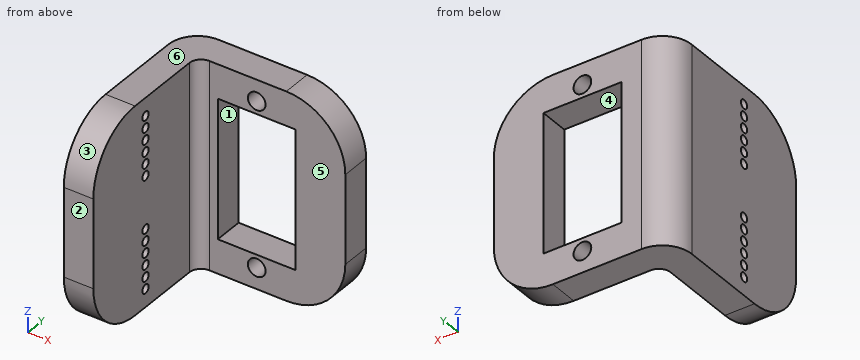
from build123d import *

# Parameters (mm, degrees)
SKETCH1_W           = 35
SKETCH1_H           = 25
SKETCH1_R           = 0.75
BOSS_EXTRUDE1_DEPTH = 5
SKETCH4_W           = 30
SKETCH4_H           = 35
BOSS_EXTRUDE2_DEPTH = 5
CUT_EXTRUDE2_REACH  = 47.894
SKETCH3_R           = 1.5
SKETCH3_W           = 23.5
SKETCH3_H           = 13.2
FILLET1_R           = 10
FILLET2_R           = 5
FILLET3_R           = 2
FILLET4_R           = 10


with BuildPart() as part:
    # Sketch1 → Boss-Extrude1 (new body)
    with BuildSketch(Plane(origin=(0, 0, 0), x_dir=(0, 0, -1), z_dir=(1, 0, 0))):
        Rectangle(SKETCH1_W, SKETCH1_H)
        with Locations((-14.45, 0)):
            Circle(SKETCH1_R, mode=Mode.SUBTRACT)
        with Locations((-12.45, 0)):
            Circle(SKETCH1_R, mode=Mode.SUBTRACT)
        with Locations((-10.45, 0)):
            Circle(SKETCH1_R, mode=Mode.SUBTRACT)
        with Locations((-8.45, 0)):
            Circle(SKETCH1_R, mode=Mode.SUBTRACT)
        with Locations((-6.45, 0)):
            Circle(SKETCH1_R, mode=Mode.SUBTRACT)
        with Locations((-4.45, 0)):
            Circle(SKETCH1_R, mode=Mode.SUBTRACT)
        with Locations((4.45, 0)):
            Circle(SKETCH1_R, mode=Mode.SUBTRACT)
        with Locations((6.45, 0)):
            Circle(SKETCH1_R, mode=Mode.SUBTRACT)
        with Locations((8.45, 0)):
            Circle(SKETCH1_R, mode=Mode.SUBTRACT)
        with Locations((10.45, 0)):
            Circle(SKETCH1_R, mode=Mode.SUBTRACT)
        with Locations((12.45, 0)):
            Circle(SKETCH1_R, mode=Mode.SUBTRACT)
        with Locations((14.45, 0)):
            Circle(SKETCH1_R, mode=Mode.SUBTRACT)
    extrude(amount=BOSS_EXTRUDE1_DEPTH)

    # Sketch4 → Boss-Extrude2 (add)
    with BuildSketch(Plane(origin=(0, 12.5, 0), x_dir=(1, 0, 0), z_dir=(0, 1, 0))):
        with Locations((15, 0)):
            Rectangle(SKETCH4_W, SKETCH4_H)
    extrude(amount=BOSS_EXTRUDE2_DEPTH)

    # Sketch3 → Cut-Extrude2 (cut, up to next)
    with BuildSketch(Plane(origin=(30, 17.5, 0), x_dir=(0, 0, -1), z_dir=(0, 1, 0)), mode=Mode.PRIVATE) as cut_extrude2_sk1:
        with Locations(Location((13.9, 15, 0), (0, 0, 180))):
            Circle(SKETCH3_R)
    cut_extrude2_tool1 = extrude(cut_extrude2_sk1.sketch, amount=-CUT_EXTRUDE2_REACH, mode=Mode.PRIVATE) & part.part
    # Sketch3 → Cut-Extrude2 (cut, up to next)
    with BuildSketch(Plane(origin=(30, 17.5, 0), x_dir=(0, 0, -1), z_dir=(0, 1, 0)), mode=Mode.PRIVATE) as cut_extrude2_sk2:
        with Locations(Location((-13.9, 15, 0), (0, 0, 180))):
            Circle(SKETCH3_R)
    cut_extrude2_tool2 = extrude(cut_extrude2_sk2.sketch, amount=-CUT_EXTRUDE2_REACH, mode=Mode.PRIVATE) & part.part
    # Sketch3 → Cut-Extrude2 (cut, up to next)
    with BuildSketch(Plane(origin=(30, 17.5, 0), x_dir=(0, 0, -1), z_dir=(0, 1, 0)), mode=Mode.PRIVATE) as cut_extrude2_sk3:
        with Locations((0, 15)):
            Rectangle(SKETCH3_W, SKETCH3_H)
    cut_extrude2_tool3 = extrude(cut_extrude2_sk3.sketch, amount=-CUT_EXTRUDE2_REACH, mode=Mode.PRIVATE) & part.part
    add(cut_extrude2_tool1.solids().sort_by_distance((15, 17.5, -13.9))[0], mode=Mode.SUBTRACT)
    add(cut_extrude2_tool2.solids().sort_by_distance((15, 17.5, 13.9))[0], mode=Mode.SUBTRACT)
    add(cut_extrude2_tool3.solids().sort_by_distance((15, 17.5, 0))[0], mode=Mode.SUBTRACT)

    # Fillet1
    fillet1_edges = [part.edges().sort_by_distance(p)[0] for p in [
        (30, 15, 17.5),
        (30, 15, -17.5),
    ]]
    fillet(fillet1_edges, radius=FILLET1_R)

    # Fillet2
    fillet2_edges = [part.edges().sort_by_distance(p)[0] for p in [
        (0, 17.5, 0),
    ]]
    fillet(fillet2_edges, radius=FILLET2_R)

    # Fillet3
    fillet3_edges = [part.edges().sort_by_distance(p)[0] for p in [
        (5, 12.5, 0),
    ]]
    fillet(fillet3_edges, radius=FILLET3_R)

    # Fillet4
    fillet4_edges = [part.edges().sort_by_distance(p)[0] for p in [
        (2.5, -12.5, -17.5),
        (2.5, -12.5, 17.5),
    ]]
    fillet(fillet4_edges, radius=FILLET4_R)


solid = part.part
Design review of the part built by this model. Coordinates are the model's own, in mm. Face numbers are marked on the shaded views. A direction names the side the tool comes from. Give positions to 0.01 mm unless a question says otherwise; leave off trailing zeros. Write each loop counter-clockwise with the first axis right and the second up, starting at its lowest first coordinate (ties: lowest second). Pieces come first, ordered by that corner, then holes. Notation, with made-up numbers: M -30,17 L -1,17 A9 ccw -1,27 Z; hole C -32,-11 d6. An arc over 180 degrees is marked long. Answer as a JSON object with one key per item and string values. Group by question number.
1) We need section D-D (y = 9.25). Give the boundary of the cut face in (x, z), and give its area (3 significant figures).
2) We need section C-C (z = 6.45). Give the boundary of the cut face in (x, y).
3) We need section A-A (z = -0.5). Give the boundary of the cut face in (x, y), and give its area (3 significant figures).
4) Mouldability with a two-part tool opening along Z and no side actions: class the marked faces 1, 2 and 3 as released by +Z, released by -Z, zero draft, split by the parting line, or undercut.
5) Tool access review of the marked faces 4, 5 and 6: name each direction out of +Z, -Z, +X, -X, +Y, -Y from which nothing blocks a thin tool from reaching the whole face with its end or side.
6) We need section B-B (x = 18.25). Give the boundary of the cut face in (y, z).
7) For line 1 along X through (y, z) = (4.25, 13.5); line 2 along Y through (x, z) = (1.9, -14.45); line 3 along Y through (x, z) = (26, -9.5), list the stretches that pass through material, from the lowest coordinate up.
8) Clearance check with flat-ended pins moving along their axes: pin 1 Ø2.5 at (y, z) = (0, 14.45) entering from +X; pin 2 Ø10 at (x, z) = (6, 0.5) entering from -Y; pin 3 Ø3.5 at (x, z) = (15, 13.9) entering from -Y. State where each tip first meets the part, or that it passes through.
Answer key:
{
 "1": {"outline": "M 0,-17.5 L 5,-17.5 L 5,17.5 L 0,17.5 Z", "area": "175 mm²"},
 "2": {"outline": "M 0,-12.5 L 5,-12.5 L 5,-0.75 L 0,-0.75 Z; M 0,0.75 L 5,0.75 L 5,10.5 A2 cw 7,12.5 L 8.4,12.5 L 8.4,17.5 L 5,17.5 A5 ccw 0,12.5 Z; M 21.6,12.5 L 30,12.5 L 30,17.5 L 21.6,17.5 Z"},
 "3": {"outline": "M 0,-12.5 L 5,-12.5 L 5,10.5 A2 cw 7,12.5 L 8.4,12.5 L 8.4,17.5 L 5,17.5 A5 ccw 0,12.5 Z; M 21.6,12.5 L 30,12.5 L 30,17.5 L 21.6,17.5 Z", "area": "204 mm²"},
 "4": {"face 1": "undercut", "face 2": "zero draft", "face 3": "released by +Z"},
 "5": {"face 4": "+Y, -Y", "face 5": "+Z, -Z, +X, -Y", "face 6": "+Z, +X, -X, +Y, -Y"},
 "6": {"outline": "M 12.5,-17.5 L 17.5,-17.5 L 17.5,-11.75 L 12.5,-11.75 Z; M 12.5,11.75 L 17.5,11.75 L 17.5,17.5 L 12.5,17.5 Z"},
 "7": {"line 1": "x = 0 to 5", "line 2": "y = -9.69 to -0.75, 0.75 to 16.42", "line 3": "y = 12.5 to 17.5"},
 "8": {"pin 1": "stops at x = 5", "pin 2": "stops at y = -12.5", "pin 3": "stops at y = 12.5"}
}
